```python
from build123d import *

# Parameters (mm, degrees)
ESQUISSE1_W             = 155
ESQUISSE1_H             = 60
ESQUISSE1_R             = 2
BOSS_EXTRU_1_DEPTH      = 18
ESQUISSE1_5_W           = 80
ESQUISSE1_5_H           = 60
ESQUISSE1_5_R           = 2
BOSS_EXTRU_2_DEPTH      = 12.5
ESQUISSE6_R             = 2
ENL_V_MAT_EXTRU_2_DEPTH = 10


with BuildPart() as part:
    # Esquisse1 → Boss.-Extru.1 (new body)
    with BuildSketch(Plane(origin=(0, 0, 0), x_dir=(0, 0, -1), z_dir=(1, 0, 0))):
        with Locations((92.673222626, -22)):
            Rectangle(ESQUISSE1_W, ESQUISSE1_H)
        with Locations((116.173222626, -38)):
            Circle(ESQUISSE1_R, mode=Mode.SUBTRACT)
        with Locations((147.173222626, -38)):
            Circle(ESQUISSE1_R, mode=Mode.SUBTRACT)
    extrude(amount=-BOSS_EXTRU_1_DEPTH)

    # Esquisse1<5> → Boss.-Extru.2 (add)
    with BuildSketch(Plane(origin=(0, 0, 0), x_dir=(0, 0, -1), z_dir=(1, 0, 0))):
        with Locations((-24.826777374, -22)):
            Rectangle(ESQUISSE1_5_W, ESQUISSE1_5_H)
        with Locations((-54.826777374, 2.55)):
            Circle(ESQUISSE1_5_R, mode=Mode.SUBTRACT)
        with Locations((5.173222626, 2.55)):
            Circle(ESQUISSE1_5_R, mode=Mode.SUBTRACT)
    extrude(amount=-BOSS_EXTRU_2_DEPTH)

    # Esquisse6 → Enlèv. mat.-Extru.2 (cut)
    with BuildSketch(Plane.XY.offset(64.826777374)):
        with Locations((-6.25, -7)):
            Circle(ESQUISSE6_R)
        with Locations((-6.25, -37)):
            Circle(ESQUISSE6_R)
    extrude(amount=-ENL_V_MAT_EXTRU_2_DEPTH, mode=Mode.SUBTRACT)


solid = part.part
```
Could you check a few things on this model? Use its own coordinates, in mm. A direction names the side the tool comes from. Give positions to 0.01 mm unless a question says otherwise; leave off trailing zeros. Order: outer loops, then holes, each group sorted by start corner. A loop starts at its lowest first (then second) coordinate and runs counter-clockwise, first axis right, second up.
Q1. If I drill on line 1 along Y through (x, z) = (-6.25, 62.5); line 2 along Z through (x, y) = (-1.75, 2.5); line 3 along X through (y, z) = (-13, 24), over which ranges is the centre line in solid material (lowest first)?
Q2. We'd pull the mould along Y, two halves only. Please class faces 4 (the flat face through (-6, -37, 54.827)), 5 (the flat face through (0, -22, -51)), 6 (the flat face through (-9, 8, -51)): +Y half, -Y half, draft (parallel to the pull), parting line (faces both ways), or undercut.
Q3. For faces 1 (the cylindrical face through (-6.684, -38.952, 59.897)), 2 (the flat face through (-12.5, -22, 25)), 3 (the cylindrical face through (-8.874, -39.952, -115.74)), which set-ups out of +Z, -Z, +X, -X, +Y, -Y let a thin tool reach every point of the face, with its end or its side?
Q4. Suppose I cut it at A-A, the plane y = -7. Write out the boundary of the cut face in (x, z).
Q5. Suppose I cut it at C-C, the plane z = 29. Write out the boundary of the cut face in (x, y).
Q6. I'm going to push flat-ended pins straight in: P1, Ø4, axis at x = -16, z = -6, coming from the +Y side; P2, Ø6, axis at y = -30, z = -10, coming from the -X side; P3, Ø1.2, axis at x = -7, y = -37, coming from the +Z side; P4, Ø3, axis at x = -16.5, y = -27.5, coming from the +Z side. Where does each tip first touch, or does it pass through?
Q7. Suppose I cut it at B-B, the plane y = 2.55. Write out the boundary of the cut face in (x, z).
Q8. Suppose I cut it at D-D, the plane y = -29. Write out the boundary of the cut face in (x, z), and give its area (3 significant figures).
Solution:
1. line 1: y = -52 to -39, -35 to -9, -5 to 8
1. line 2: z = -170.17 to -7.17, -3.17 to 52.83, 56.83 to 64.83
1. line 3: x = -12.5 to 0
2. face 4: undercut
2. face 5: draft
2. face 6: +Y half
3. face 1: +Z
3. face 2: +Z, -X, +Y, -Y
3. face 3: +X, -X
4. outline: (-18, -170.17) - (0, -170.17) - (0, 64.83) - (-4.25, 64.83) - (-4.25, 54.83) - (-8.25, 54.83) - (-8.25, 64.83) - (-12.5, 64.83) - (-12.5, -15.17) - (-18, -15.17) - close
5. outline: (-12.5, -52) - (0, -52) - (0, 8) - (-12.5, 8) - close
6. P1: passes through
6. P2: stops at x = -12.5
6. P3: stops at z = 54.83
6. P4: stops at z = -15.17
7. outline: (-18, -170.17) - (0, -170.17) - (0, -7.17) - (-12.5, -7.17) - (-12.5, -15.17) - (-18, -15.17) - close; (-12.5, -3.17) - (0, -3.17) - (0, 52.83) - (-12.5, 52.83) - close; (-12.5, 56.83) - (0, 56.83) - (0, 64.83) - (-12.5, 64.83) - close
8. outline: (-18, -170.17) - (0, -170.17) - (0, 64.83) - (-12.5, 64.83) - (-12.5, -15.17) - (-18, -15.17) - close
8. area: 3,790 mm2
